Model file for the job. Use its own axes, mm. Face numbers are marked on the shaded views. A direction names the side the tool comes from. Round coordinates to 2 decimals unless told otherwise and drop trailing zeros. Loops run counter-clockwise (first coordinate to the right, second up) from the corner with the lowest first, then second, coordinate; pieces in that order, holes last. Notation, with made-up numbers: (-6, 43.5) - (29, 43.5) arc R13 ccw to (29, 48.5) - close; hole circle Ø2 at (68.5, 54). An arc over 180 degrees is marked (long way). Answer as a JSON object with one key per item and string values.
from build123d import *

# Parameters (mm, degrees)
SKETCH1_R           = 6.35
BOSS_EXTRUDE1_DEPTH = 63.5
CIRPATTERN1_COUNT   = 2
CIRPATTERN1_ANGLE   = 90


with BuildPart() as part:
    # Sketch1 → Boss-Extrude1 (new body)
    with BuildSketch(Plane.XY):
        Circle(SKETCH1_R)
    boss_extrude1 = extrude(amount=BOSS_EXTRUDE1_DEPTH)

    # CirPattern1: Boss-Extrude1 ×2 about axis
    cirpattern1_axis = Axis((0, 6.35, 31.75), (0, -1, 0))
    for i in range(1, CIRPATTERN1_COUNT):
        add(boss_extrude1.rotate(cirpattern1_axis, i * CIRPATTERN1_ANGLE / (CIRPATTERN1_COUNT - 1)))


solid = part.part
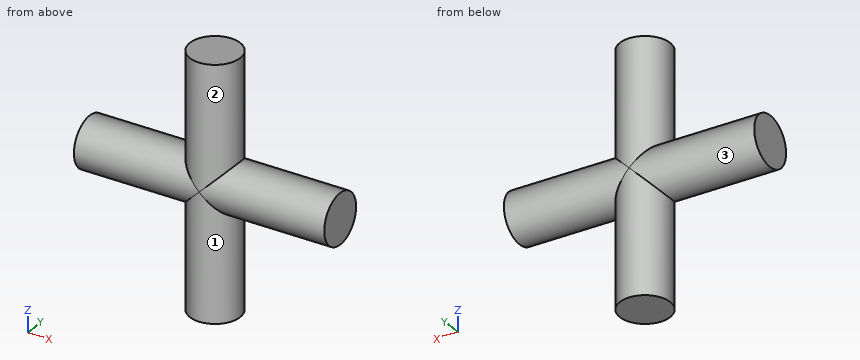
1) Slice it at D-D on y = -4.25. List the corners of the cut face in (x, z), then the cut area to 3 significant figures.
Values follow:
{"outline": "(-31.75, 27.03) - (-4.72, 27.03) - (-4.72, 0) - (4.72, 0) - (4.72, 27.03) - (31.75, 27.03) - (31.75, 36.47) - (4.72, 36.47) - (4.72, 63.5) - (-4.72, 63.5) - (-4.72, 36.47) - (-31.75, 36.47) - close", "area": "1,110 mm²"}
2) Slice it at B-B on x = -3. List the corners of the cut face in (y, z).
Values follow:
{"outline": "(-5.6, 0) - (5.6, 0) - (5.6, 28.75) arc R6.35 ccw to (5.6, 34.75) - (5.6, 63.5) - (-5.6, 63.5) - (-5.6, 34.75) arc R6.35 ccw to (-5.6, 28.75) - close"}
3) Drop flat-ended pins along their axis: P1, Ø4, axis at x = 3.5, z = 23, coming from the -Y side; P2, Ø1, axis at x = 17, y = 1, coming from the +Z side; P3, Ø3, axis at x = -17.5, z = 37.5, coming from the -Y side. Give the stop position or say it passes through.
Values follow:
{"P1": "y = -6.17", "P2": "z = 38.08", "P3": "y = -4.72"}
4) Probe probe 1 along X at (y, z) = (1.75, 53.5); probe 2 along Z at (x, y) = (-19, -3); probe 3 along Y at (x, z) = (-4.5, 41). List the from-to ranges inside material, lowest first.
Values follow:
{"probe 1": "-6.1 to 6.1", "probe 2": "26.15 to 37.35", "probe 3": "-4.48 to 4.48"}
5) Slice it at A-A on y = 0. List the corners of the cut face in (x, z), then the cut area to 3 significant figures.
Values follow:
{"outline": "(-31.75, 25.4) - (-6.35, 25.4) - (-6.35, 0) - (6.35, 0) - (6.35, 25.4) - (31.75, 25.4) - (31.75, 38.1) - (6.35, 38.1) - (6.35, 63.5) - (-6.35, 63.5) - (-6.35, 38.1) - (-31.75, 38.1) - close", "area": "1,450 mm²"}
6) Slice it at C-C on z = 8.5. List the corners of the cut face in (x, y).
Values follow:
{"outline": "circle Ø12.7 at (0, 0)"}
7) Tool access for the marked faces 1, 2 and 3: list every direction of +Z, -Z, +X, -X, +Y, -Y with a clear straight run to the whole face (end or side of a thin tool).
Values follow:
{"face 1": "-Z", "face 2": "+Z", "face 3": "-X"}
